Input: dimensioned drawing with shaded views. Units: mm. Origin: part minimum x, y, z. Round coordinates to 2 decimals unless told otherwise and drop trailing zeros. Loops run counter-clockwise (first coordinate to the right, second up) from the corner with the lowest first, then second, coordinate; pieces in that order, holes last. Notation, with made-up numbers: (24, 50.25) - (66, 50.25) arc R22 ccw to (66, 68.25) - close; hole circle Ø8 at (-7, 70.5). An arc over 180 degrees is marked (long way). Answer as CSV lines item,"result".
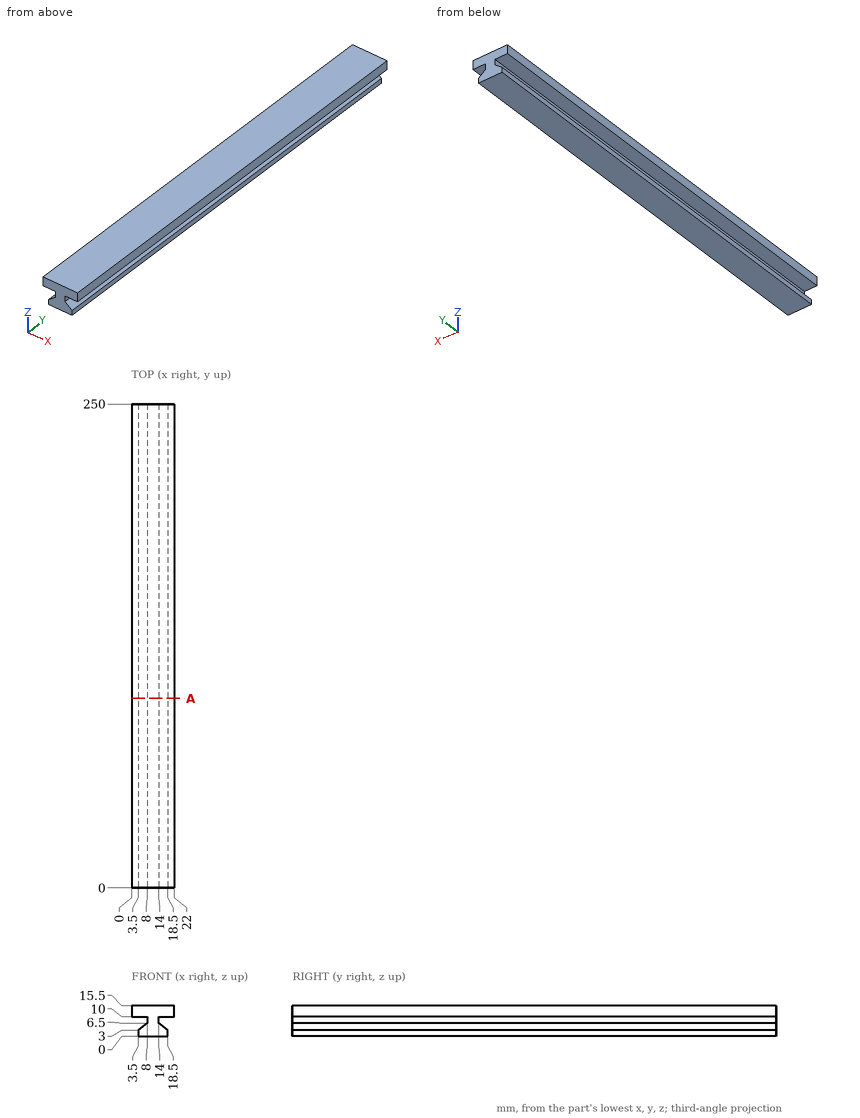
(1) Material intervals for line 1 along Z through (x, y) = (19.75, 46); line 2 along X through (y, z) = (216.5, 0.75); line 3 along Z through (x, y) = (7.25, 205), sorted ascending.
Findings below:
line 1,"10 to 15.5"
line 2,"3.5 to 18.5"
line 3,"0 to 5.92, 10 to 15.5"
(2) Pin query (flat end, axial travel): P1, Ø2, axis at y = 219.5, z = 2.5, coming from the +X side; P2, Ø1, axis at y = 174.5, z = 9, coming from the -X side; P3, Ø0.9, axis at y = 178, z = 2, coming from the -X side. Return the tip coordinate at first contact, or that it passes through.
Findings below:
P1,"x = 18.5"
P2,"x = 8"
P3,"x = 3.5"
(3) Section A-A (y = 98). Output: boundary loops of the cut face in (x, z).
Findings below:
outline,"(0, 10) - (8, 10) - (8, 6.5) - (3.5, 3) - (3.5, 0) - (18.5, 0) - (18.5, 3) - (14, 6.5) - (14, 10) - (22, 10) - (22, 15.5) - (0, 15.5) - close"
